Verification items for this drawing (mm, ordinates from the low corner). Give positions to 0.01 mm unless a question says otherwise; leave off trailing zeros. Loops run counter-clockwise (first coordinate to the right, second up) from the corner with the lowest first, then second, coordinate; pieces in that order, holes last. Notation, with made-up numbers: M 26,-9.75 L 57,-9.75 A8 cw 57,-4.75 Z; hole C -39.5,-28 d10. An arc over 180 degrees is marked long. Put each result on its own line as item: value. Start each with the question number.
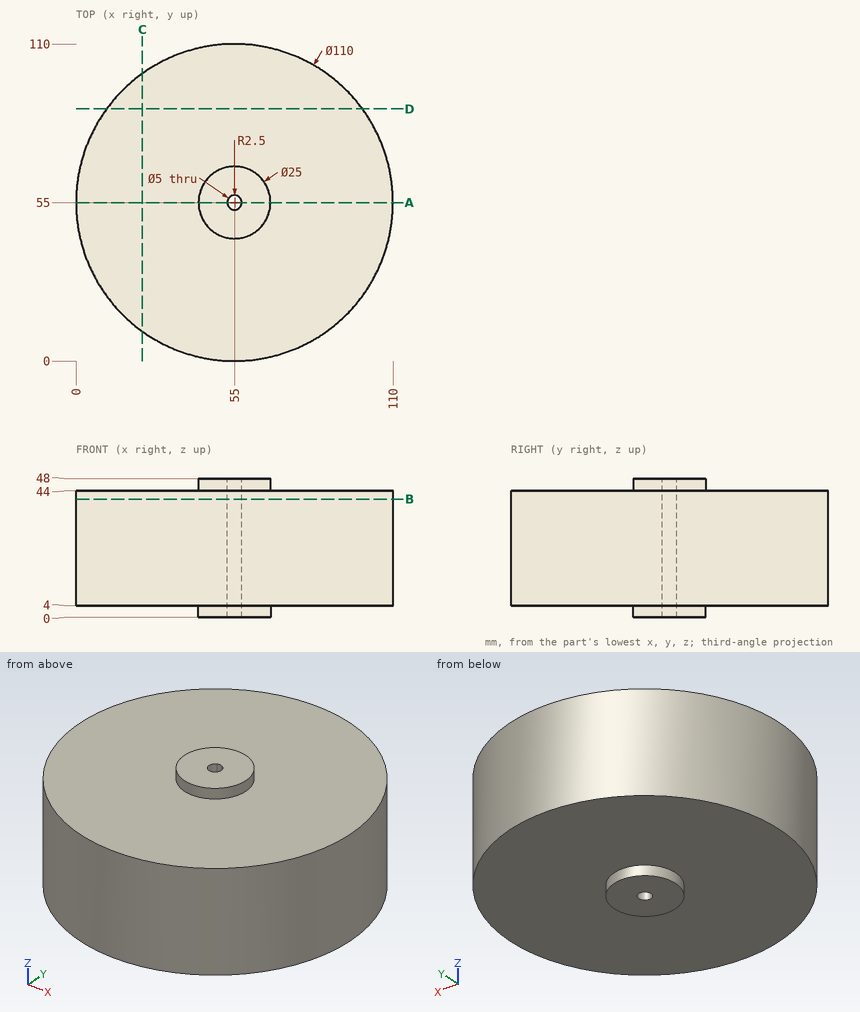
Q1. Cross-section at A-A, the plane y = 55. Record the boundary of the cut face in (x, z).
Q2. Go/stop test with flat-tipped pins: pin 1 (12 mm diameter, centred on y = 30.5, z = 42, fed in from -X); pin 2 (6 mm diameter, centred on y = 29, z = 28, fed in from -X); pin 3 (8 mm diameter, centred on x = 96, y = 29.5, fed in from -Z); pin 4 (4 mm diameter, centred on x = 55, y = 55, fed in from +Z). Record where each tip stops, or that it passes through.
Q3. Cross-section at C-C, the plane x = 23. Record the boundary of the cut face in (y, z).
Q4. Cross-section at D-D, the plane y = 87.5. Record the boundary of the cut face in (x, z), then the cut area to 3 significant figures.
Q5. Cross-section at B-B, the plane z = 41. Record the boundary of the cut face in (x, y), then the cut area to 3 significant figures.
Q6. Scan lines: L1, parallel to Y at x = 55, z = 36; L2, parallel to Z at x = 54.5, y = 103; L3, parallel to Y at x = 53, z = 39.5. Record each from-to range of solid material in increasing order.
Ans:
1. outline: M 0,4 L 42.5,4 L 42.5,0 L 52.5,0 L 52.5,48 L 42.5,48 L 42.5,44 L 0,44 Z; M 57.5,0 L 67.5,0 L 67.5,4 L 110,4 L 110,44 L 67.5,44 L 67.5,48 L 57.5,48 Z
2. pin 1: stops at x = 3.2
2. pin 2: stops at x = 5.04
2. pin 3: stops at z = 4
2. pin 4: passes through
3. outline: M 10.27,4 L 99.73,4 L 99.73,44 L 10.27,44 Z
4. outline: M 10.63,4 L 99.37,4 L 99.37,44 L 10.63,44 Z
4. area: 3,550 mm^2
5. outline: C 55,55 d110; hole C 55,55 d5
5. area: 9,480 mm^2
6. L1: y = 0 to 52.5, 57.5 to 110
6. L2: z = 4 to 44
6. L3: y = 0.04 to 53.5, 56.5 to 109.96
